Part model, mm, in its own coordinate system. A direction names the side the tool comes from. Give positions to 0.01 mm unless a question says otherwise; leave off trailing zeros. Write each loop counter-clockwise with the first axis right and the second up, starting at its lowest first coordinate (ties: lowest second). Pieces come first, ordered by that corner, then holes.
Autodesk Inventor part; units mm, degrees
ref_plane "YZ Plane" through (0, 0, 0) normal (1, 0, 0) x (0, 1, 0)
ref_plane "XZ Plane" through (0, 0, 0) normal (0, 1, 0) x (-1, 0, 0)
ref_plane "XY Plane" through (0, 0, 0) normal (0, 0, 1) x (1, 0, 0)
sketch "Sketch1" plane through (0, 0, 0) normal (1, 0, 0) x (0, 1, 0)
  line L0 (0, 9.525) -> (-63.5, 9.525)
  line L1 (-63.5, 9.525) -> (-63.5, -9.525)
  line L2 (-63.5, -9.525) -> (0, -9.525)
  line L3 (0, -9.525) -> (0, 9.525)
  arc A0 (0, -9.525) -> (0, 9.525) centre (0, 0) ccw
  dimension "d0" = 19.05
  dimension "d1" = 63.5
extrude "Extrusion1" add sketch "Sketch1" along normal blind 12.7
sketch "Sketch3" plane through (12.7, 0, 0) normal (1, 0, 0) x (0, 0, -1)
  line L0 (-9.525, 0) -> (-9.525, -63.5)
  line L1 (-9.525, -63.5) -> (9.525, -63.5)
  line L2 (9.525, -63.5) -> (9.525, 0)
  arc A0 (9.525, 0) -> (-9.525, 0) centre (0, 0) ccw
  line L3 (-6.35, -63.5) -> (6.35, -63.5)
  line L4 (6.35, -63.5) -> (6.35, -38.1)
  line L5 (6.35, -38.1) -> (-6.35, -38.1)
  line L6 (-6.35, -38.1) -> (-6.35, -63.5)
  point P0 (0, -63.5)
  dimension "d18" = 12.7
  dimension "d19" = 6.35
  dimension "d20" = 25.4
extrude "Extrusion3" cut sketch "Sketch3" against normal blind 6.35 contours L6 L5 L4 L1
sketch "Sketch4" plane through (12.7, 0, 0) normal (1, 0, 0) x (0, 0, -1)
  line L0 (-6.35, -63.5) -> (-6.35, -38.1)
  line L1 (-6.35, -38.1) -> (6.35, -38.1)
  line L2 (6.35, -38.1) -> (6.35, -63.5)
  line L3 (6.35, -63.5) -> (9.525, -63.5)
  line L4 (9.525, -63.5) -> (9.525, 0)
  arc A0 (9.525, 0) -> (-9.525, 0) centre (0, 0) ccw
  line L5 (-9.525, 0) -> (-9.525, -63.5)
  line L6 (-9.525, -63.5) -> (-6.35, -63.5)
  circle A1 centre (0, 0) radius 9.525
  line L7 (-14.2875, 12.7) -> (12.7, 12.7)
  line L8 (12.7, 12.7) -> (12.7, -4.7625)
  line L9 (12.7, -4.7625) -> (-14.2875, -4.7625)
  line L10 (-14.2875, -4.7625) -> (-14.2875, 12.7)
  point P0 (-8.2489, -4.7625)
  point P1 (-9.525, 0)
  point P2 (9.525, 0)
  point P3 (8.2489, -4.7625)
  dimension "d28" = 19.05
extrude "Extrusion4" [suppressed]
sketch "Sketch5" plane through (12.7, 0, 0) normal (1, 0, 0) x (0, 0, -1)
  arc A0 (1.8331, 11.9745) -> (-1.9, 11.7198) centre (0, 11.3568) ccw
  line L0 (-1.9, 11.7198) -> (-4, 0.7283)
  arc A1 (-5.4371, -0.709) -> (-4, 0.7283) centre (-5.4371, 0.7281) ccw
  line L1 (-5.4371, -0.709) -> (-16.4286, -2.8088)
  arc A2 (-16.4286, -2.8088) -> (-16.4286, -6.6088) centre (-16.0656, -4.7088) ccw
  line L2 (-16.4286, -6.6088) -> (-5.4371, -8.7087)
  arc A3 (-4, -10.146) -> (-5.4371, -8.7087) centre (-5.4371, -10.1458) ccw
  line L3 (-4, -10.146) -> (-1.9, -21.1375)
  arc A4 (-1.9, -21.1375) -> (1.9, -21.1375) centre (0, -20.7745) ccw
  line L4 (1.9, -21.1375) -> (4, -10.146)
  arc A5 (5.4371, -8.7088) -> (4, -10.146) centre (5.4371, -10.146) ccw
  line L5 (5.4371, -8.7088) -> (16.4286, -6.6088)
  arc A6 (16.4286, -6.6088) -> (16.4286, -2.8088) centre (16.0656, -4.7088) ccw
  line L6 (16.4286, -2.8088) -> (5.4367, -0.7088)
  arc A7 (4.0053, 0.6052) -> (5.4367, -0.7088) centre (5.4371, 0.7283) ccw
  line L7 (4.0053, 0.6052) -> (1.8331, 11.9745)
  line L8 (-6.35, -63.5) -> (-6.35, -38.1)
  line L9 (-6.35, -38.1) -> (6.35, -38.1)
  line L10 (6.35, -38.1) -> (6.35, -63.5)
  line L11 (6.35, -63.5) -> (9.525, -63.5)
  line L12 (9.525, -63.5) -> (9.525, 0)
  arc A8 (9.525, 0) -> (-9.525, 0) centre (0, 0) ccw
  line L13 (-9.525, 0) -> (-9.525, -63.5)
  line L14 (-9.525, -63.5) -> (-6.35, -63.5)
  line L15 (-4.509, 0.7712) -> (-2.399, 11.8152)
  arc A9 (2.3259, 12.1019) -> (-2.399, 11.8152) centre (0, 11.3568) ccw
  line L16 (2.3259, 12.1019) -> (4.5097, 0.672)
  arc A10 (4.5097, 0.672) -> (5.4797, -0.1998) centre (5.4371, 0.7283) ccw
  line L17 (5.4797, -0.1998) -> (16.524, -2.3098)
  arc A11 (16.524, -7.1078) -> (16.524, -2.3098) centre (16.0656, -4.7088) ccw
  line L18 (16.524, -7.1078) -> (5.48, -9.2178)
  arc A12 (5.48, -9.2178) -> (4.509, -10.1889) centre (5.4371, -10.146) ccw
  line L19 (4.509, -10.1889) -> (2.399, -21.2328)
  arc A13 (-2.399, -21.2328) -> (2.399, -21.2328) centre (0, -20.7745) ccw
  line L20 (-2.399, -21.2328) -> (-4.509, -10.1888)
  arc A14 (-4.509, -10.1888) -> (-5.48, -9.2177) centre (-5.4371, -10.1458) ccw
  line L21 (-5.48, -9.2177) -> (-16.524, -7.1078)
  arc A15 (-16.524, -2.3098) -> (-16.524, -7.1078) centre (-16.0656, -4.7088) ccw
  line L22 (-16.524, -2.3098) -> (-5.48, -0.2)
  arc A16 (-5.48, -0.2) -> (-4.509, 0.7712) centre (-5.4371, 0.7281) ccw
  circle A17 centre (0, -4.7088) radius 19.5082
  point P0 (2.905, 9.0712)
  point P1 (9.525, -0.9727)
  point P2 (9.525, -8.445)
  point P3 (9.525, -21.7336)
  point P4 (-9.525, -21.7336)
  point P5 (-9.525, -8.4449)
  point P6 (-9.525, -0.9728)
  point P7 (-2.9244, 9.065)
  dimension "d29" = 0
  dimension "d30" = 0.508
extrude "Extrusion5" add sketch "Sketch5" against normal up to surface (12.7 mm away) contours L7 A8 L0 A0 | A0 L0 A8 L15 A9 L16 L7 | A8 L16 A10 L17 L12 L6 A7 L7 | L7 A7 L6 L12 L5 A5 L4 A4 L3 A3 L2 L13 L1 A1 L0 A8 | L0 A1 L1 L13 L22 A16 L15 A8 | L16 A9 L15 A8 L13 L22 A15 L21 A17 L12 L18 A11 L17 | L12 L17 A11 L18 L5 A6 L6 | L6 A6 L5 L12 | L13 L2 A2 L1 | L1 A2 L2 L13 L21 A15 L22 | L12 L18 A12 L19 A13 L20 A14 L21 L13 L2 A3 L3 A4 L4 A5 L5
extrude "Extrusion6" cut sketch "Sketch5" against normal blind 9.525 contours L7 A8 L0 A0 | A0 L0 A8 L15 A9 L16 L7 | A8 L16 A10 L17 L12 L6 A7 L7 | L7 A7 L6 L12 L5 A5 L4 A4 L3 A3 L2 L13 L1 A1 L0 A8 | L0 A1 L1 L13 L22 A16 L15 A8 | L12 L17 A11 L18 L5 A6 L6 | L6 A6 L5 L12 | L13 L2 A2 L1 | L1 A2 L2 L13 L21 A15 L22 | L12 L18 A12 L19 A13 L20 A14 L21 L13 L2 A3 L3 A4 L4 A5 L5
properties part number "Part_3_hand"
1) 3-axis set-ups, long thin cutter, end or side, ignore diameter. For faces 4 (the flat face through (10, -51, 6.35)), 5 (the cylindrical face through (8.004, -4.662, 18.508)), 6 (the flat face through (12.7, -16, -4)), 7 (the flat face through (6, -43, -9.525)), 8 (the flat face through (5, -63.5, 0)): which of +Z, -Z, +X, -X, +Y, -Y reach the whole face in a straight line?
Check result:
face 4: +X, -Y
face 5: +X
face 6: +Z, -Z, +X, +Y, -Y
face 7: -Z, +X, -X, -Y
face 8: +Z, -Z, +X, -X, -Y
2) Mould opens along Y. For faces 1 (the flat face through (6, -42, 9.525)), 2 (the flat face through (8, -1.24, -10.92)), 3 (the cylindrical face through (6.439, 14.786, -0.719)) say: +Y half, -Y half, draft (parallel to the pull), parting line (faces both ways), or undercut.
Check result:
face 1: draft
face 2: undercut
face 3: parting line
3) Saw through at B-B (y = -43.5). Write the cut outline in (x, z) (3 decimals), and give its area (3 significant figures).
Check result:
outline: (0, -9.525) - (12.7, -9.525) - (12.7, -6.35) - (6.35, -6.35) - (6.35, 6.35) - (12.7, 6.35) - (12.7, 9.525) - (0, 9.525) - close
area: 161 mm2
4) Saw through at D-D (x = 1.5). Write the cut outline in (y, z) (3 decimals).
Check result:
outline: (-63.5, -9.525) - (-21.734, -9.525) arc R19.508 ccw (long way) to (-21.734, 9.525) - (-63.5, 9.525) - close
5) Saw through at C-C (z = 0). Write the cut outline in (x, y) (3 decimals).
Check result:
outline: (0, -63.5) - (6.35, -63.5) - (6.35, -38.1) - (12.7, -38.1) - (12.7, -23.217) - (3.175, -23.217) - (3.175, 13.799) - (12.7, 13.799) - (12.7, 14.799) - (0, 14.799) - close
6) Flat gauge pins, fed straight in: P1, Ø1.5, axis at x = 6, y = -53, coming from the +Z side (3 decimals); P2, Ø5, axis at x = 10.5, z = 1, coming from the -Y side; P3, Ø1, axis at x = 11, y = -17.5, coming from the +Z side. Where does each tip first touch, or does it go through?
Check result:
P1: stops at z = 9.525
P2: stops at y = -38.1
P3: stops at z = 15.15
7) Drill centre lines: L1, parallel to Z at x = 6, y = -2.5; L2, parallel to Y at x = 5, z = -8; L3, parallel to Y at x = 11.25, z = 14.5. Where is each one in solid material? Low to high.
Check result:
L1: z = -19.38 to -17.11, 17.11 to 19.38
L2: y = -63.5 to -8.74, -0.68 to 13.08
L3: y = -17.76 to -7.49, -1.92 to 8.34
